The model under review builds one solid part; all positions refer to its coordinate system, in mm. A direction names the side the tool comes from. Round coordinates to 2 decimals unless told otherwise and drop trailing zeros. Order: outer loops, then holes, each group sorted by start corner. A loop starts at its lowest first (then second) coordinate and runs counter-clockwise, first axis right, second up. Notation, with made-up numbers: M 28.5,-27 L 61.5,-27 A14 cw 61.5,0 Z; hole C 48,24.25 d2. An arc over 180 degrees is marked long. One line per item, written item: value. Start each with the question number.
from build123d import *

# Parameters (mm, degrees)
SKETCH1_W           = 160.3375
SKETCH1_H           = 611.1875
BOSS_EXTRUDE1_DEPTH = 5.588
FILLET1_R           = 3.175
SKETCH2_R           = 4.7625
CUT_EXTRUDE1_DEPTH  = 6.35
SKETCH3_W           = 76.2
SKETCH3_H           = 25.4
CUT_EXTRUDE2_DEPTH  = 6.35
FILLET2_R           = 3.175
FILLET3_R           = 12.7
SKETCH4_R           = 2.38125
CUT_EXTRUDE3_DEPTH  = 25.4


with BuildPart() as part:
    # Sketch1 → Boss-Extrude1 (new body)
    with BuildSketch(Plane(origin=(0, 0, 0), x_dir=(1, 0, 0), z_dir=(0, 1, 0))):
        Rectangle(SKETCH1_W, SKETCH1_H)
    extrude(amount=BOSS_EXTRUDE1_DEPTH)

    # Fillet1
    fillet1_edges = [part.edges().sort_by_distance(p)[0] for p in [
        (80.16875, 2.794, 305.59375),
        (-80.16875, 2.794, 305.59375),
        (-80.16875, 2.794, -305.59375),
        (80.16875, 2.794, -305.59375),
    ]]
    fillet(fillet1_edges, radius=FILLET1_R)

    # Sketch2 → Cut-Extrude1 (cut)
    with BuildSketch(Plane(origin=(0, 5.588, 0), x_dir=(1, 0, 0), z_dir=(0, 1, 0))):
        with Locations(Location((62.70625, 245.26875, 0), (0, 0, 270))):
            Circle(SKETCH2_R)
        with Locations(Location((-64.29375, 245.26875, 0), (0, 0, 270))):
            Circle(SKETCH2_R)
        with Locations(Location((-64.29375, -288.13125, 0), (0, 0, 270))):
            Circle(SKETCH2_R)
    extrude(amount=-CUT_EXTRUDE1_DEPTH, mode=Mode.SUBTRACT)

    # Sketch3 → Cut-Extrude2 (cut)
    with BuildSketch(Plane(origin=(0, 5.588, 0), x_dir=(1, 0, 0), z_dir=(0, 1, 0))):
        with Locations((15.875, -292.89375)):
            Rectangle(SKETCH3_W, SKETCH3_H)
    extrude(amount=-CUT_EXTRUDE2_DEPTH, mode=Mode.SUBTRACT)

    # Fillet2
    fillet2_edges = [part.edges().sort_by_distance(p)[0] for p in [
        (-22.225, 2.794, 305.59375),
        (53.975, 2.794, 305.59375),
    ]]
    fillet(fillet2_edges, radius=FILLET2_R)

    # Fillet3
    fillet3_edges = [part.edges().sort_by_distance(p)[0] for p in [
        (-22.225, 2.794, 280.19375),
        (53.975, 2.794, 280.19375),
    ]]
    fillet(fillet3_edges, radius=FILLET3_R)

    # Sketch4 → Cut-Extrude3 (cut)
    with BuildSketch(Plane(origin=(0, 5.588, 0), x_dir=(1, 0, 0), z_dir=(0, 1, 0))):
        with Locations(Location((-40.29075, 203.99375, 0), (0, 0, 270))):
            Circle(SKETCH4_R)
        with Locations(Location((-40.29075, 153.95575, 0), (0, 0, 270))):
            Circle(SKETCH4_R)
        with Locations(Location((51.745051389, 203.99375, 0), (0, 0, 270))):
            Circle(SKETCH4_R)
        with Locations(Location((50.89525, 153.95575, 0), (0, 0, 270))):
            Circle(SKETCH4_R)
        with BuildLine():
            Line((-26.63825, 203.99375), (42.839342829, 203.99375))
            ThreePointArc((42.839342829, 203.99375), (44.635394053, 203.249801224), (45.379342829, 201.45375))
            Line((45.379342829, 201.45375), (45.379342829, 158.115))
            ThreePointArc((45.379342829, 158.115), (44.635394053, 156.318948776), (42.839342829, 155.575))
            Line((42.839342829, 155.575), (-26.63825, 155.575))
            ThreePointArc((-26.63825, 155.575), (-28.434301224, 156.318948776), (-29.17825, 158.115))
            Line((-29.17825, 158.115), (-29.17825, 201.45375))
            ThreePointArc((-29.17825, 201.45375), (-28.434301224, 203.249801224), (-26.63825, 203.99375))
        make_face()
    extrude(amount=-CUT_EXTRUDE3_DEPTH, mode=Mode.SUBTRACT)


solid = part.part
Item 1: Clearance check with flat-ended pins moving along their axes: P1, Ø4.5, axis at x = -40.29, z = -203.99, coming from the +Y side; P2, Ø1.7, axis at x = 11.5, y = 2, coming from the +Z side. State where each tip first meets the part, or that it passes through.
Item 2: Consider section A-A, the plane z = -170. Give the boundary of the cut face in (x, y), then the cut area to 3 significant figures.
Item 3: Consider section B-B, the plane x = -16. Give the boundary of the cut face in (y, z) (3 decimals).
Item 4: Consider section C-C, the plane y = 3.7. Count the separate pieces of the cut face and the enclosed holes in it, then the cut area to 3 significant figures.
Item 5: Machinability: for faces 1 (the flat face through (-1, 5.588, -4)), 2 (the cylindrical face through (-18.41, 2.75, 283.82)), which of the approach directions +Z, -Z, +X, -X, +Y, -Y give a long, thin tool a straight path to every point of the face, cutting with its end or side? Answer none if there is none.
Item 6: Wall thickness on L1, parallel to Z at x = 40, y = 0.7 (3 decimals); L2, parallel to Z at x = -27.5, y = 0.5: over which ranges is each line inside the solid? List them lowest first.
Computed:
1. P1: passes through
1. P2: stops at z = 280.19
2. outline: M -80.17,0 L -29.18,0 L -29.18,5.59 L -80.17,5.59 Z; M 45.38,0 L 80.17,0 L 80.17,5.59 L 45.38,5.59 Z
2. area: 479 mm^2
3. outline: M 0,-305.594 L 5.588,-305.594 L 5.588,-203.994 L 0,-203.994 Z; M 0,-155.575 L 5.588,-155.575 L 5.588,281.968 L 0,281.968 Z
4. separate pieces: 1
4. enclosed holes: 8
4. area: 92,200 mm^2
5. face 1: +Z, -Z, +X, -X, +Y
5. face 2: +Z, +Y, -Y
6. L1: z = -305.594 to -203.994, -155.575 to 280.194
6. L2: z = -305.59 to -203.84, -155.73 to 305.59
